Work out the finished part from the listing and answer in its coordinate system (mm). A direction names the side the tool comes from. Give positions to 0.01 mm unless a question says otherwise; leave off trailing zeros. Write each loop counter-clockwise with the first axis right and the second up, starting at its lowest first coordinate (ties: lowest second). Pieces come first, ordered by that corner, then holes. Notation, with made-up numbers: (28, 19) - (78, 19) arc R22 ccw to (78, 26) - close; hole circle Ø3 at (-22.75, -1). An arc over 180 degrees is marked (long way). Write item = value, one per line.
from build123d import *

# Parameters (mm, degrees)
EXTRUDE_1_DEPTH = 30


with BuildPart() as part:
    # 草圖1 → 擠出1 (new, symmetric)
    with BuildSketch(Plane.XY):
        with BuildLine():
            Line((-15, -3.25), (-12.5, -3.25))
            Line((-12.5, -3.25), (-12.5, -5.072439755))
            Line((-12.5, -5.072439755), (-6.47547695, -5.072439755))
            ThreePointArc((-6.47547695, -5.072439755), (-4.5, 0), (-6.47547695, 5.072439755))
            Line((-6.47547695, 5.072439755), (-12.5, 5.072439755))
            Line((-12.5, 5.072439755), (-12.5, 3.25))
            Line((-12.5, 3.25), (-15, 3.25))
            Line((-15, 3.25), (-15, 15))
            Line((-15, 15), (-3.25, 15))
            Line((-3.25, 15), (-3.25, 12.5))
            Line((-3.25, 12.5), (-5.25, 12.5))
            Line((-5.25, 12.5), (-5.25, 6.643928679))
            ThreePointArc((-5.25, 6.643928679), (0, 4.5), (5.25, 6.643928679))
            Line((5.25, 6.643928679), (5.25, 12.5))
            Line((5.25, 12.5), (3.25, 12.5))
            Line((3.25, 12.5), (3.25, 15))
            Line((3.25, 15), (15, 15))
            Line((15, 15), (15, 3.25))
            Line((15, 3.25), (12.5, 3.25))
            Line((12.5, 3.25), (12.5, 5.072439755))
            Line((12.5, 5.072439755), (6.47547695, 5.072439755))
            ThreePointArc((6.47547695, 5.072439755), (4.5, 0), (6.47547695, -5.072439755))
            Line((6.47547695, -5.072439755), (12.5, -5.072439755))
            Line((12.5, -5.072439755), (12.5, -3.25))
            Line((12.5, -3.25), (15, -3.25))
            Line((15, -3.25), (15, -15))
            Line((15, -15), (3.25, -15))
            Line((3.25, -15), (3.25, -12.5))
            Line((3.25, -12.5), (5.25, -12.5))
            Line((5.25, -12.5), (5.25, -6.643928679))
            ThreePointArc((5.25, -6.643928679), (0, -4.5), (-5.25, -6.643928679))
            Line((-5.25, -6.643928679), (-5.25, -12.5))
            Line((-5.25, -12.5), (-3.25, -12.5))
            Line((-3.25, -12.5), (-3.25, -15))
            Line((-3.25, -15), (-15, -15))
            Line((-15, -15), (-15, -3.25))
        make_face()
        with BuildLine():
            Line((-9.25, -6.072439755), (-6.25, -6.072439755))
            Line((-6.25, -6.072439755), (-6.25, -9.25))
            Line((-6.25, -9.25), (-7.09526249, -9.25))
            ThreePointArc((-7.09526249, -9.25), (-7, -10), (-7.09526249, -10.75))
            Line((-7.09526249, -10.75), (-6.75, -10.75))
            ThreePointArc((-6.75, -10.75), (-6.396446609, -10.896446609), (-6.25, -11.25))
            Line((-6.25, -11.25), (-6.25, -14))
            Line((-6.25, -14), (-9.25, -14))
            Line((-9.25, -14), (-9.25, -12.90473751))
            ThreePointArc((-9.25, -12.90473751), (-10, -13), (-10.75, -12.90473751))
            Line((-10.75, -12.90473751), (-10.75, -14))
            Line((-10.75, -14), (-14, -14))
            Line((-14, -14), (-14, -10.786219878))
            Line((-14, -10.786219878), (-12.895143918, -10.786219878))
            ThreePointArc((-12.895143918, -10.786219878), (-12.999766765, -10.037407923), (-12.913849333, -9.286219878))
            Line((-12.913849333, -9.286219878), (-14, -9.286219878))
            Line((-14, -9.286219878), (-14, -6.072439755))
            Line((-14, -6.072439755), (-10.75, -6.072439755))
            Line((-10.75, -6.072439755), (-10.75, -7.09526249))
            ThreePointArc((-10.75, -7.09526249), (-10, -7), (-9.25, -7.09526249))
            Line((-9.25, -7.09526249), (-9.25, -6.072439755))
        make_face(mode=Mode.SUBTRACT)
        with BuildLine():
            Line((-14, 6.072439755), (-10.75, 6.072439755))
            Line((-10.75, 6.072439755), (-10.75, 7.09526249))
            ThreePointArc((-10.75, 7.09526249), (-10, 7), (-9.25, 7.09526249))
            Line((-9.25, 7.09526249), (-9.25, 6.072439755))
            Line((-9.25, 6.072439755), (-6.25, 6.072439755))
            Line((-6.25, 6.072439755), (-6.25, 9.25))
            Line((-6.25, 9.25), (-7.09526249, 9.25))
            ThreePointArc((-7.09526249, 9.25), (-7, 10), (-7.09526249, 10.75))
            Line((-7.09526249, 10.75), (-6.75, 10.75))
            ThreePointArc((-6.75, 10.75), (-6.396446609, 10.896446609), (-6.25, 11.25))
            Line((-6.25, 11.25), (-6.25, 14))
            Line((-6.25, 14), (-9.25, 14))
            Line((-9.25, 14), (-9.25, 12.90473751))
            ThreePointArc((-9.25, 12.90473751), (-10, 13), (-10.75, 12.90473751))
            Line((-10.75, 12.90473751), (-10.75, 14))
            Line((-10.75, 14), (-14, 14))
            Line((-14, 14), (-14, 10.786219878))
            Line((-14, 10.786219878), (-12.895143918, 10.786219878))
            ThreePointArc((-12.895143918, 10.786219878), (-12.999766765, 10.037407923), (-12.913849333, 9.286219878))
            Line((-12.913849333, 9.286219878), (-14, 9.286219878))
            Line((-14, 9.286219878), (-14, 6.072439755))
        make_face(mode=Mode.SUBTRACT)
        with BuildLine():
            Line((14, 14), (14, 10.786219878))
            Line((14, 10.786219878), (12.895143918, 10.786219878))
            ThreePointArc((12.895143918, 10.786219878), (12.999766765, 10.037407923), (12.913849333, 9.286219878))
            Line((12.913849333, 9.286219878), (14, 9.286219878))
            Line((14, 9.286219878), (14, 6.072439755))
            Line((14, 6.072439755), (10.75, 6.072439755))
            Line((10.75, 6.072439755), (10.75, 7.09526249))
            ThreePointArc((10.75, 7.09526249), (10, 7), (9.25, 7.09526249))
            Line((9.25, 7.09526249), (9.25, 6.072439755))
            Line((9.25, 6.072439755), (6.25, 6.072439755))
            Line((6.25, 6.072439755), (6.25, 9.25))
            Line((6.25, 9.25), (7.09526249, 9.25))
            ThreePointArc((7.09526249, 9.25), (7, 10), (7.09526249, 10.75))
            Line((7.09526249, 10.75), (6.75, 10.75))
            ThreePointArc((6.75, 10.75), (6.396446609, 10.896446609), (6.25, 11.25))
            Line((6.25, 11.25), (6.25, 14))
            Line((6.25, 14), (9.25, 14))
            Line((9.25, 14), (9.25, 12.90473751))
            ThreePointArc((9.25, 12.90473751), (10, 13), (10.75, 12.90473751))
            Line((10.75, 12.90473751), (10.75, 14))
            Line((10.75, 14), (14, 14))
        make_face(mode=Mode.SUBTRACT)
        with BuildLine():
            Line((7.09526249, -10.75), (6.75, -10.75))
            ThreePointArc((6.75, -10.75), (6.396446609, -10.896446609), (6.25, -11.25))
            Line((6.25, -11.25), (6.25, -14))
            Line((6.25, -14), (9.25, -14))
            Line((9.25, -14), (9.25, -12.90473751))
            ThreePointArc((9.25, -12.90473751), (10, -13), (10.75, -12.90473751))
            Line((10.75, -12.90473751), (10.75, -14))
            Line((10.75, -14), (14, -14))
            Line((14, -14), (14, -10.786219878))
            Line((14, -10.786219878), (12.895143918, -10.786219878))
            ThreePointArc((12.895143918, -10.786219878), (12.999766765, -10.037407923), (12.913849333, -9.286219878))
            Line((12.913849333, -9.286219878), (14, -9.286219878))
            Line((14, -9.286219878), (14, -6.072439755))
            Line((14, -6.072439755), (10.75, -6.072439755))
            Line((10.75, -6.072439755), (10.75, -7.09526249))
            ThreePointArc((10.75, -7.09526249), (10, -7), (9.25, -7.09526249))
            Line((9.25, -7.09526249), (9.25, -6.072439755))
            Line((9.25, -6.072439755), (6.25, -6.072439755))
            Line((6.25, -6.072439755), (6.25, -9.25))
            Line((6.25, -9.25), (7.09526249, -9.25))
            ThreePointArc((7.09526249, -9.25), (7, -10), (7.09526249, -10.75))
        make_face(mode=Mode.SUBTRACT)
        with BuildLine():
            ThreePointArc((3.948754255, 3.296580342), (3.537868444, 2.020477551), (3.327916667, 0.696398348))
            ThreePointArc((3.327916667, 0.696398348), (3.4, 0), (3.327916667, -0.696398348))
            ThreePointArc((3.327916667, -0.696398348), (3.537868444, -2.020477551), (3.948754255, -3.296580342))
            ThreePointArc((3.948754255, -3.296580342), (3.839592373, -3.839592373), (3.296580342, -3.948754255))
            ThreePointArc((3.296580342, -3.948754255), (2.020477551, -3.537868444), (0.696398348, -3.327916667))
            ThreePointArc((0.696398348, -3.327916667), (0, -3.4), (-0.696398348, -3.327916667))
            ThreePointArc((-0.696398348, -3.327916667), (-2.020477551, -3.537868444), (-3.296580342, -3.948754255))
            ThreePointArc((-3.296580342, -3.948754255), (-3.839592373, -3.839592373), (-3.948754255, -3.296580342))
            ThreePointArc((-3.948754255, -3.296580342), (-3.537868444, -2.020477551), (-3.327916667, -0.696398348))
            ThreePointArc((-3.327916667, -0.696398348), (-3.4, 0), (-3.327916667, 0.696398348))
            ThreePointArc((-3.327916667, 0.696398348), (-3.537868444, 2.020477551), (-3.948754255, 3.296580342))
            ThreePointArc((-3.948754255, 3.296580342), (-3.839592373, 3.839592373), (-3.296580342, 3.948754255))
            ThreePointArc((-3.296580342, 3.948754255), (-2.020477551, 3.537868444), (-0.696398348, 3.327916667))
            ThreePointArc((-0.696398348, 3.327916667), (0, 3.4), (0.696398348, 3.327916667))
            ThreePointArc((0.696398348, 3.327916667), (2.020477551, 3.537868444), (3.296580342, 3.948754255))
            ThreePointArc((3.296580342, 3.948754255), (3.839592373, 3.839592373), (3.948754255, 3.296580342))
        make_face(mode=Mode.SUBTRACT)
    extrude(amount=EXTRUDE_1_DEPTH, both=True)


solid = part.part
1. Straight lines are drawn through the part: line 1 (Y direction, x = 13.5, z = -10.5); line 2 (X direction, y = 10.25, z = 26); line 3 (Y direction, x = 7.25, z = -21.5). For each, find the intervals that lie inside material, in ascending order.
Solution:
line_1 = -15 to -14, -10.79 to -9.29, -6.07 to -3.25, 3.25 to 6.07, 9.29 to 10.79, 14 to 15
line_2 = -15 to -12.99, -7.01 to -5.25, 5.25 to 7.01, 12.99 to 15
line_3 = -15 to -14, -6.07 to -5.07, 5.07 to 6.07, 14 to 15
2. For a pull along X with two mould halves and no side action, classify faces 3 (the flat face through (12.5, -4, 0)), 4 (the flat face through (-14, -3.25, 0)), 5 (the flat face through (15, -9, 0)) as pulls with the +X half, pulls with the -X half, needs draft (parallel to the pull), parting line crosses it, or undercut.
Solution:
face_3 = undercut
face_4 = needs draft
face_5 = pulls with the +X half
3. Find section A-A, the plane x = 1.75. Give the vertices of the cut face in (y, z).
Solution:
outline = (-4.71, -30) - (-3.48, -30) - (-3.48, 30) - (-4.71, 30) - close; (3.48, -30) - (4.71, -30) - (4.71, 30) - (3.48, 30) - close
4. Find section C-C, the plane y = 1.5. Give the vertices of the cut face in (x, z).
Solution:
outline = (-4.65, -30) - (-3.43, -30) - (-3.43, 30) - (-4.65, 30) - close; (3.43, -30) - (4.65, -30) - (4.65, 30) - (3.43, 30) - close
5. Find section B-B, the plane z = 22. Give the number of separate pieces and of enclosed holes in the cut face, then the cut area to 3 significant figures.
Solution:
separate_pieces = 1
enclosed_holes = 5
area = 257 mm^2
6. A tool of negligible diameter and unlimited length cuts with its end or side. For faces 1 (the flat face through (14, 12, 0)), 2 (the flat face through (-4, 0, -30)), from which of +Z, -Z, +X, -X, +Y, -Y can it reach the whole face along a straight path? Write none if from no direction.
Solution:
face_1 = +Z, -Z
face_2 = -Z, +X, -X, +Y, -Y
